The listing builds one solid part. Answer for the finished solid, in the listing's coordinates (mm). A direction names the side the tool comes from. Round coordinates to 2 decimals unless told otherwise and drop trailing zeros. Loops run counter-clockwise (first coordinate to the right, second up) from the corner with the lowest first, then second, coordinate; pieces in that order, holes last. Notation, with made-up numbers: (3, -10) -> (23, -10) arc R26 cw to (23, 27) -> close; hole circle Ø2 at (80, 8.25). An arc over 180 degrees is marked (long way). Use a Markdown table: item, result. Add a question column.
Q1. Consider line 1 (Z direction, x = 0, y = -17); line 2 (Z direction, x = 7.5, y = -13.25); line 3 (Z direction, x = -7, y = -23.75). Determine where each line is inside the solid, lowest interval first.
Q2. Section B-B on z = -10 is taken. Give the vertices of the cut face in (x, y), then the cut area to 3 significant figures.
Q3. Which of the six approach directions +Z, -Z, +X, -X, +Y, -Y give full straight-line access (tool end or side, diameter ignored) to faces 4 (the flat face through (-23.9, -13, -30)), 5 (the flat face through (-15, -15.3, -24.93)), 6 (the cylindrical face through (-17.77, -13.68, -29.8)), 7 (the flat face through (23.9, -13, -30)), 8 (the flat face through (15.2, -15.3, -24.93))?
Q4. Section A-A on y = -9 is taken. Give the vertices of the cut face in (x, z), then the cut area to 3 significant figures.
Q5. Section C-C on y = -21 is taken. Give the vertices of the cut face in (x, z), then the cut area to 3 significant figures.
Q6. Given pin 1 Ø9.5 at (x, y) = (14.7, -10.86) entering from -Z; pin 2 Ø22.5 at (x, z) = (0, 0) entering from -Y; pin 3 Ø3.5 at (y, z) = (-8.5, -23) entering from -X; pin 4 Ø10 at (y, z) = (-9.5, -8.5) entering from +X, each flat-ended and moving along its own axis, determine where each tip first touches the part or whether it passes through.
Q7. Section D-D on x = 13 is taken. Give the vertices of the cut face in (y, z).
Q8. For a pull along Z with two mould halves and no side action, classify faces 1 (the flat face through (0, -13, -34.545)), 2 (the flat face through (-6.35, -13, -21)), 3 (the flat face through (0, 0, -19)) as released by +Z, released by -Z, zero draft, split by the parting line, or undercut.
from build123d import *

# Parameters (mm, degrees)
F1_DEPTH = 25.4
F2_R     = 4.1683581246
F3_DEPTH = 10.668


# Not quite as in the source:
# - a feature names something its author has since deleted; it is built from what else it names


with BuildPart() as f1:
    # F0 (on Front) → F1 (new body)
    with BuildSketch(Plane.XZ):
        with BuildLine():
            ThreePointArc((6.35, -18.0951603751), (11.0901618338, 15.6449876798), (-19.177, 0))
            ThreePointArc((-19.177, 0), (-15.6449876798, -11.0901618338), (-6.35, -18.0951603751))
            Line((-6.35, -18.0951603751), (-6.35, -24.9301567674))
            Line((-6.35, -24.9301567674), (-23.899981752, -24.9301567674))
            Line((-23.899981752, -24.9301567674), (-23.899981752, -34.5450900495))
            Line((-23.899981752, -34.5450900495), (23.899981752, -34.5450900495))
            Line((23.899981752, -34.5450900495), (23.899981752, -24.9301567674))
            Line((23.899981752, -24.9301567674), (6.35, -24.9301567674))
            Line((6.35, -24.9301567674), (6.35, -18.0951603751))
        make_face()
        with BuildLine():
            ThreePointArc((-14.097, 0), (0, 14.097), (14.097, 0))
            ThreePointArc((14.097, 0), (0, -14.097), (-14.097, 0))
        make_face(mode=Mode.SUBTRACT)
    extrude(amount=F1_DEPTH)

    # F2 (on face) → F3 (cut)
    with BuildSketch(Plane(origin=(0, 0, -34.5450900495), x_dir=(1, 0, 0), z_dir=(0, 0, -1))):
        with Locations((-14.7024132311, 10.8604691923)):
            Circle(F2_R)
        with Locations((14.7024132311, 10.8604691923)):
            Circle(F2_R)
    extrude(amount=-F3_DEPTH, mode=Mode.SUBTRACT)


solid = f1.part
Checked values:
| question | item | result |
|---|---|---|
| 1 | line 1 | z = -34.55 to -14.1, 14.1 to 19.18 |
| 1 | line 2 | z = -34.55 to -24.93, -17.65 to -11.94, 11.94 to 17.65 |
| 1 | line 3 | z = -34.55 to -24.93, -17.85 to -12.24, 12.24 to 17.85 |
| 2 | outline | (-16.36, -25.4) -> (-9.94, -25.4) -> (-9.94, 0) -> (-16.36, 0) -> close; (9.94, -25.4) -> (16.36, -25.4) -> (16.36, 0) -> (9.94, 0) -> close |
| 2 | area | 327 mm2 |
| 3 | face 4 | +Z, -Z, -X, +Y, -Y |
| 3 | face 5 | -X, +Y, -Y |
| 3 | face 6 | -Z |
| 3 | face 7 | +Z, -Z, +X, +Y, -Y |
| 3 | face 8 | +X, +Y, -Y |
| 4 | outline | (-23.9, -34.55) -> (-18.43, -34.55) -> (-18.43, -24.93) -> (-23.9, -24.93) -> close; (-10.97, -34.55) -> (10.97, -34.55) -> (10.97, -24.93) -> (6.35, -24.93) -> (6.35, -18.1) arc R19.18 ccw (long way) to (-6.35, -18.1) -> (-6.35, -24.93) -> (-10.97, -24.93) -> close; (18.43, -34.55) -> (23.9, -34.55) -> (23.9, -24.93) -> (18.43, -24.93) -> close; hole circle Ø28.19 at (0, 0) |
| 4 | area | 925 mm2 |
| 5 | outline | (-23.9, -34.55) -> (23.9, -34.55) -> (23.9, -24.93) -> (6.35, -24.93) -> (6.35, -18.1) arc R19.18 ccw (long way) to (-6.35, -18.1) -> (-6.35, -24.93) -> (-23.9, -24.93) -> close; hole circle Ø28.19 at (0, 0) |
| 5 | area | 1,070 mm2 |
| 6 | pin 1 | stops at z = -34.55 |
| 6 | pin 2 | passes through |
| 6 | pin 3 | stops at x = -6.35 |
| 6 | pin 4 | stops at x = 18.85 |
| 7 | outline | (-25.4, -34.55) -> (-14.67, -34.55) -> (-14.67, -24.93) -> (-25.4, -24.93) -> close; (-25.4, -14.1) -> (0, -14.1) -> (0, -5.45) -> (-25.4, -5.45) -> close; (-25.4, 5.45) -> (0, 5.45) -> (0, 14.1) -> (-25.4, 14.1) -> close; (-7.06, -34.55) -> (0, -34.55) -> (0, -24.93) -> (-7.06, -24.93) -> close |
| 8 | face 1 | released by -Z |
| 8 | face 2 | undercut |
| 8 | face 3 | zero draft |
